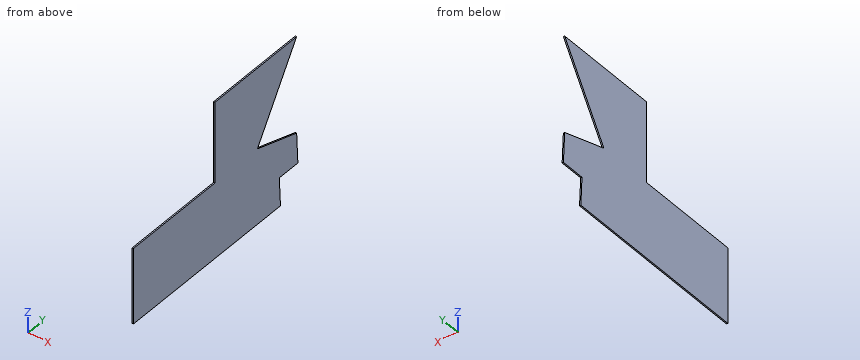
Autodesk Inventor part; units mm, degrees
ref_plane "YZ Plane" through (0, 0, 0) normal (1, 0, 0) x (0, 1, 0)
ref_plane "XZ Plane" through (0, 0, 0) normal (0, 1, 0) x (-1, 0, 0)
ref_plane "XY Plane" through (0, 0, 0) normal (0, 0, 1) x (1, 0, 0)
sketch "Sketch1" plane through (0, 0, 0) normal (1, 0, 0) x (0, 1, 0)
  line L0 (0, 0) -> (-698.5, 0)
  line L1 (-698.5, 0) -> (-698.5, 381)
  line L2 (-698.5, 381) -> (0, 381)
  line L3 (0, 381) -> (0, 0)
  line L4 (-444.5, 381) -> (-444.5, 184.15)
  line L5 (-444.5, 184.15) -> (-698.5, 184.15)
  line L6 (-189.3272, 381) -> (-311.7065, 184.15)
  line L7 (-311.7065, 184.15) -> (-189.3272, 145.8189)
  line L8 (-189.3272, 145.8189) -> (-185.4527, 70.4)
  line L9 (-185.4527, 70.4) -> (-243.3711, 70.4)
  line L10 (-243.3711, 70.4) -> (-239.7544, 0)
  dimension "d0" = 698.5
  dimension "d1" = 381
  dimension "d3" = 254
  dimension "d4" = 196.85
extrude "Plate1" add sketch "Sketch1" along normal blind 3.175 contours L0 L1 L5 L4 L2 L6 L7 L8 L9 L10
equation "\"d2\" = Thickness"
equation "\"BendRadius\" = Thickness"
equation "\"BendReliefWidth\" = Thickness"
equation "\"BendReliefDepth\" = 0.5 * Thickness"
equation "\"CornerReliefSize\" = 4 * Thickness"
equation "\"MinimumRemnant\" = 2 * Thickness"
equation "\"TransitionRadius\" = BendRadius"
equation "\"JacobiRadiusSize\" = BendRadius"
equation "\"GapSize\" = Thickness"
properties part number "PLATE,HOPPER,BACK2" material "Polycarbonate, Clear"
Geometry check sheet. Reference: the model listing, model coordinates, mm. Coordinates: 2 decimals unless noted, no trailing zeros. Write each loop counter-clockwise with the first axis right and the second up, starting at its lowest first coordinate (ties: lowest second). Pieces come first, ordered by that corner, then holes. Notation, with made-up numbers: M -27.5,4.25 L 21.5,4.25 A19 cw 21.5,37.25 Z; hole C 26.25,48.5 d5. An arc over 180 degrees is marked long. Answer as a JSON object with one key per item and string values.
1. Section check B-B, the plane x = 2.2. Enter the section's corners in (y, z).
Answers below:
{"outline": "M -698.5,0 L -239.75,0 L -243.37,70.4 L -185.45,70.4 L -189.33,145.82 L -311.71,184.15 L -189.33,381 L -444.5,381 L -444.5,184.15 L -698.5,184.15 Z"}
2. Scan lines: L1, parallel to Z at x = 0.9, y = -533.5; L2, parallel to Z at x = 1.8, y = -245; L3, parallel to Z at x = 1.15, y = -295. Record each from-to range of solid material in increasing order.
Answers below:
{"L1": "z = 0 to 184.15", "L2": "z = 0 to 163.26, 291.45 to 381", "L3": "z = 0 to 178.92, 211.02 to 381"}
3. Section check A-A, the plane y = -306. Enter the section's corners in (x, z) (3 decimals), plus the area to 3 significant figures.
Answers below:
{"outline": "M 0,0 L 3.175,0 L 3.175,182.363 L 0,182.363 Z; M 0,193.329 L 3.175,193.329 L 3.175,381 L 0,381 Z", "area": "1,170 mm²"}
4. Section check C-C, the plane y = -535. Enter the section's corners in (x, z) (3 decimals).
Answers below:
{"outline": "M 0,0 L 3.175,0 L 3.175,184.15 L 0,184.15 Z"}
5. Section check D-D, the plane z = 158.5. Enter the section's corners in (x, y) (3 decimals).
Answers below:
{"outline": "M 0,-698.5 L 3.175,-698.5 L 3.175,-229.814 L 0,-229.814 Z"}
